Geometry check sheet. Reference: the model listing, model coordinates, mm. Face numbers are marked on the shaded views. A direction names the side the tool comes from. Round coordinates to 2 decimals unless told otherwise and drop trailing zeros. Loops run counter-clockwise (first coordinate to the right, second up) from the corner with the lowest first, then second, coordinate; pieces in that order, holes last. Notation, with made-up numbers: M 23,-19 L 42,-19 A27 cw 42,14 Z; hole C 51,78 d7. An arc over 180 degrees is marked long. Write item = value, one per line.
from build123d import *

# Parameters (mm, degrees)
F1_DEPTH = 41.5
F2_R     = 1.5
F3_DEPTH = 103


with BuildPart() as f1:
    # F0 (on Top) → F1 (new body)
    with BuildSketch(Plane.XY):
        with BuildLine():
            Line((51.7, 45.2), (-51.4, 45.2))
            ThreePointArc((-51.4, 45.2), (-55.9961940777, 43.2961940777), (-57.9, 38.7))
            Line((-57.9, 38.7), (-57.9, -38.7))
            ThreePointArc((-57.9, -38.7), (-55.9961940777, -43.2961940777), (-51.4, -45.2))
            Line((-51.4, -45.2), (51.7, -45.2))
            ThreePointArc((51.7, -45.2), (56.2961940777, -43.2961940777), (58.2, -38.7))
            Line((58.2, -38.7), (58.2, 38.7))
            ThreePointArc((58.2, 38.7), (56.2961940777, 43.2961940777), (51.7, 45.2))
        make_face()
        with BuildLine():
            Line((-54.7, -19.5394540004), (-54.7, 18.7))
            ThreePointArc((-54.7, 18.7), (-53.2355339059, 22.2355339059), (-49.7, 23.7))
            Line((-49.7, 23.7), (-49.3605459996, 23.7))
            ThreePointArc((-49.3605459996, 23.7), (-46.4185957098, 24.9185957098), (-45.2, 27.8605459996))
            Line((-45.2, 27.8605459996), (-45.2, 37))
            ThreePointArc((-45.2, 37), (-43.7355339059, 40.5355339059), (-40.2, 42))
            Line((-40.2, 42), (40.5, 42))
            ThreePointArc((40.5, 42), (44.0355339059, 40.5355339059), (45.5, 37))
            Line((45.5, 37), (45.5, 27.8605459996))
            ThreePointArc((45.5, 27.8605459996), (46.7185957098, 24.9185957098), (49.6605459996, 23.7))
            Line((49.6605459996, 23.7), (50.8394540004, 23.7))
            ThreePointArc((50.8394540004, 23.7), (53.7814042902, 22.4814042902), (55, 19.5394540004))
            Line((55, 19.5394540004), (55, -19.5394540004))
            ThreePointArc((55, -19.5394540004), (53.7814042902, -22.4814042902), (50.8394540004, -23.7))
            Line((50.8394540004, -23.7), (49.6605459996, -23.7))
            ThreePointArc((49.6605459996, -23.7), (46.7185957098, -24.9185957098), (45.5, -27.8605459996))
            Line((45.5, -27.8605459996), (45.5, -37))
            ThreePointArc((45.5, -37), (44.0355339059, -40.5355339059), (40.5, -42))
            Line((40.5, -42), (-40.2, -42))
            ThreePointArc((-40.2, -42), (-43.7355339059, -40.5355339059), (-45.2, -37))
            Line((-45.2, -37), (-45.2, -27.8605459996))
            ThreePointArc((-45.2, -27.8605459996), (-46.4185957098, -24.9185957098), (-49.3605459996, -23.7))
            Line((-49.3605459996, -23.7), (-50.5394540004, -23.7))
            ThreePointArc((-50.5394540004, -23.7), (-53.4814042902, -22.4814042902), (-54.7, -19.5394540004))
        make_face(mode=Mode.SUBTRACT)
    extrude(amount=F1_DEPTH)

    # F2 (on Front) → F3 (cut)
    with BuildSketch(Plane.XZ):
        with Locations((-30.9, 34.73)):
            Circle(F2_R)
        with BuildLine():
            ThreePointArc((32.7, 34.7302867395), (31.1998566303, 36.2302867326), (29.7000000274, 34.73))
            Line((29.7000000274, 34.73), (32.6999999726, 34.73))
            ThreePointArc((32.6999999726, 34.73), (32.6999999931, 34.7301433697), (32.7, 34.7302867395))
        make_face()
        with BuildLine():
            Line((32.6999999726, 34.73), (29.7000000274, 34.73))
            ThreePointArc((29.7000000274, 34.73), (31.2, 33.2302867395), (32.6999999726, 34.73))
        make_face()
        with BuildLine():
            ThreePointArc((12, 34.8408361703), (10.4445440024, 36.3398106972), (9.0041004902, 34.73))
            Line((9.0041004902, 34.73), (11.9958995098, 34.73))
            ThreePointArc((11.9958995098, 34.73), (11.9989745269, 34.7853801727), (12, 34.8408361703))
        make_face()
        with BuildLine():
            Line((11.9958995098, 34.73), (9.0041004902, 34.73))
            ThreePointArc((9.0041004902, 34.73), (10.5, 33.3408361703), (11.9958995098, 34.73))
        make_face()
        with BuildLine():
            ThreePointArc((-8.7, 34.8408361703), (-10.2554559976, 36.3398106972), (-11.6958995098, 34.73))
            Line((-11.6958995098, 34.73), (-8.7041004902, 34.73))
            ThreePointArc((-8.7041004902, 34.73), (-8.7010254731, 34.7853801727), (-8.7, 34.8408361703))
        make_face()
        with BuildLine():
            Line((-8.7041004902, 34.73), (-11.6958995098, 34.73))
            ThreePointArc((-11.6958995098, 34.73), (-10.2, 33.3408361703), (-8.7041004902, 34.73))
        make_face()
        with Locations((-30.9, 9.8)):
            Circle(F2_R)
        with Locations((31.2, 9.9408361703)):
            Circle(F2_R)
        with Locations((10.5, 9.9408361703)):
            Circle(F2_R)
        with Locations((-10.2, 9.9408361703)):
            Circle(F2_R)
        with BuildLine():
            Line((-35.1, 28.9438347778), (-35.1, 15.5561652222))
            ThreePointArc((-35.1, 15.5561652222), (-34.2195334956, 13.6516675833), (-32.1983109948, 13.0886470474))
            Line((-32.1983109948, 13.0886470474), (-28.7983109948, 13.6421354195))
            ThreePointArc((-28.7983109948, 13.6421354195), (-27.2955023611, 14.4901200986), (-26.7, 16.1096535943))
            Line((-26.7, 16.1096535943), (-26.7, 28.3903464057))
            ThreePointArc((-26.7, 28.3903464057), (-27.2955023611, 30.0098799014), (-28.7983109948, 30.8578645805))
            Line((-28.7983109948, 30.8578645805), (-32.1983109948, 31.4113529526))
            ThreePointArc((-32.1983109948, 31.4113529526), (-34.2195334956, 30.8483324167), (-35.1, 28.9438347778))
        make_face()
        with BuildLine():
            Line((-14.4, 28.9788489457), (-14.4, 15.5511510543))
            ThreePointArc((-14.4, 15.5511510543), (-13.5159372403, 13.6436010981), (-11.4890025317, 13.0851662447))
            Line((-11.4890025317, 13.0851662447), (-8.0890025317, 13.6518329114))
            ThreePointArc((-8.0890025317, 13.6518329114), (-6.5924500438, 14.5018804806), (-6, 16.117817721))
            Line((-6, 16.117817721), (-6, 28.412182279))
            ThreePointArc((-6, 28.412182279), (-6.5924500438, 30.0281195194), (-8.0890025317, 30.8781670886))
            Line((-8.0890025317, 30.8781670886), (-11.4890025317, 31.4448337553))
            ThreePointArc((-11.4890025317, 31.4448337553), (-13.5159372403, 30.8863989019), (-14.4, 28.9788489457))
        make_face()
        with BuildLine():
            Line((6.3, 28.9729987336), (6.3, 15.5570012664))
            ThreePointArc((6.3, 15.5570012664), (7.1859263693, 13.6478741584), (9.2158130517, 13.0918238882))
            Line((9.2158130517, 13.0918238882), (12.5158130517, 13.6484503943))
            ThreePointArc((12.5158130517, 13.6484503943), (14.009127108, 14.4995541418), (14.6, 16.1136277725))
            Line((14.6, 16.1136277725), (14.6, 28.4163722275))
            ThreePointArc((14.6, 28.4163722275), (14.009127108, 30.0304458582), (12.5158130517, 30.8815496057))
            Line((12.5158130517, 30.8815496057), (9.2158130517, 31.4381761118))
            ThreePointArc((9.2158130517, 31.4381761118), (7.1859263693, 30.8821258416), (6.3, 28.9729987336))
        make_face()
        with BuildLine():
            Line((27, 28.9788489457), (27, 15.5511510543))
            ThreePointArc((27, 15.5511510543), (27.8840627597, 13.6436010981), (29.9109974683, 13.0851662447))
            Line((29.9109974683, 13.0851662447), (33.3109974683, 13.6518329114))
            ThreePointArc((33.3109974683, 13.6518329114), (34.8075499562, 14.5018804806), (35.4, 16.117817721))
            Line((35.4, 16.117817721), (35.4, 28.412182279))
            ThreePointArc((35.4, 28.412182279), (34.8075499562, 30.0281195194), (33.3109974683, 30.8781670886))
            Line((33.3109974683, 30.8781670886), (29.9109974683, 31.4448337553))
            ThreePointArc((29.9109974683, 31.4448337553), (27.8840627597, 30.8863989019), (27, 28.9788489457))
        make_face()
    extrude(amount=F3_DEPTH, mode=Mode.SUBTRACT)


solid = f1.part
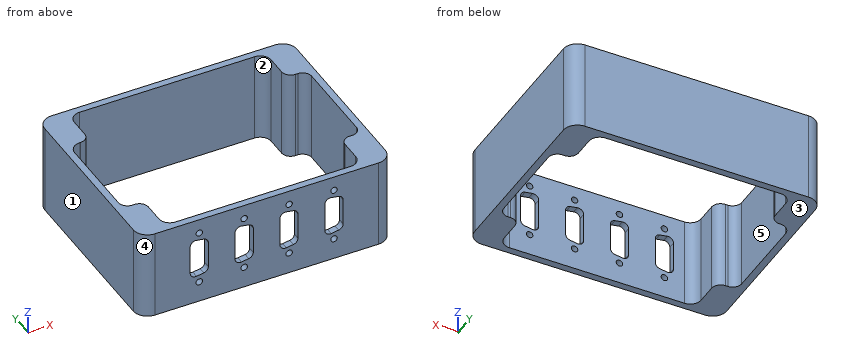
(1) Tool access check on the marked faces 4 and 5. Record the directions out of +Z, -Z, +X, -X, +Y, -Y that give a thin tool (end or side, any length) a straight path to the whole face; none if there is none.
Result set:
face_4 = +Z, -Z, -X, -Y
face_5 = +Z, -Z
(2) Sectioned sample at B-B on y = -1.5. Record the cut outline in (x, z), then the cut area to 3 significant figures.
Result set:
outline = M -57.9,0 L -54.7,0 L -54.7,41.5 L -57.9,41.5 Z; M 55,0 L 58.2,0 L 58.2,41.5 L 55,41.5 Z
area = 266 mm2
(3) Sectioned sample at A-A on x = -30.9. Record the cut outline in (y, z), then the cut area to 3 significant figures.
Result set:
outline = M -45.2,0 L -42,0 L -42,8.3 L -45.2,8.3 Z; M -45.2,11.3 L -42,11.3 L -42,13.3 L -45.2,13.3 Z; M -45.2,31.2 L -42,31.2 L -42,33.23 L -45.2,33.23 Z; M -45.2,36.23 L -42,36.23 L -42,41.5 L -45.2,41.5 Z; M 42,0 L 45.2,0 L 45.2,41.5 L 42,41.5 Z
area = 189 mm2
(4) Sectioned sample at D-D on x = 2. Record the cut outline in (y, z).
Result set:
outline = M -45.2,0 L -42,0 L -42,41.5 L -45.2,41.5 Z; M 42,0 L 45.2,0 L 45.2,41.5 L 42,41.5 Z
(5) Depth check by flat-ended pin: pin 1 Ø1.8 at (x, z) = (-30.9, 9.8) entering from -Y; pin 2 Ø3.5 at (y, z) = (-43, 20.5) entering from -X; pin 3 Ø1 at (y, z) = (-43, 20.5) entering from +X. Enter the tip coordinate at first touch or a pass-through.
Result set:
pin_1 = 42
pin_2 = -57.38
pin_3 = 56.97
(6) Release check for a two-part mould opening along X. For the marked faces 1, 2 and 3 record: released by +X, released by -X, zero draft, split by the parting line, or undercut.
Result set:
face_1 = released by -X
face_2 = undercut
face_3 = zero draft
(7) Material ranges on line 1 along Y through (x, z) = (49.5, 16); line 2 along Y through (x, z) = (2, 22.5); line 3 along X through (y, z) = (19, 17.5), recorded low to high. Write a range as from..to.
Result set:
line_1 = -45.2..-23.7, 23.7..45.2
line_2 = -45.2..-42, 42..45.2
line_3 = -57.9..-54.69, 55..58.2
